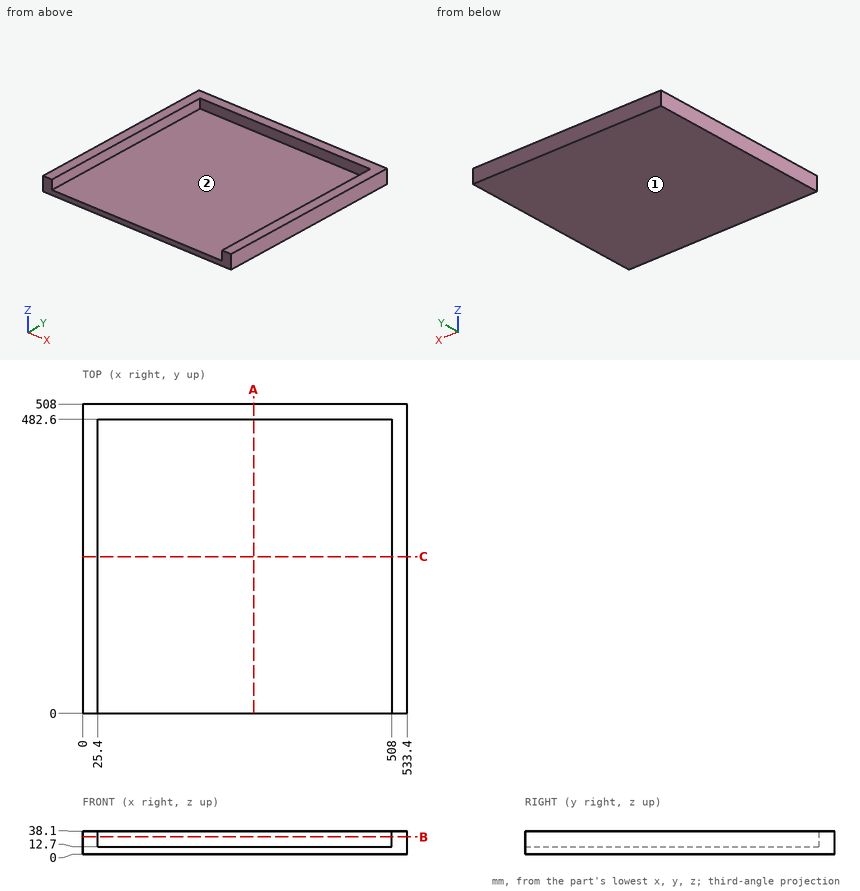
Here's the drawing with two shaded views (mm, measured from the low corner). I have some questions. Coordinates: 2 decimals unless noted, no trailing zeros. Write each loop counter-clockwise with the first axis right and the second up, starting at its lowest first coordinate (ties: lowest second). Pieces come first, ordered by that corner, then holes. Notation, with made-up numbers: (57.25, 67.25) -> (67.25, 67.25) arc R4 cw to (67.25, 71.25) -> close; hole circle Ø11 at (17, 79). An arc over 180 degrees is marked (long way). Answer as CSV lines item,"result".
1) If we section it at A-A on x = 281: Please give me the cut outline in (y, z), then the cut area to 3 significant figures.
Check result:
outline,"(0, 0) -> (508, 0) -> (508, 38.1) -> (482.6, 38.1) -> (482.6, 12.7) -> (0, 12.7) -> close"
area,"7,100 mm²"
2) If I drill on line 1 (X direction, y = 461.5, z = 28.5); line 2 (Z direction, x = 501.5, y = 338.5); line 3 (Y direction, x = 246, z = 21), over which ranges is the centre line in solid material (lowest first)? Write a range as from..to.
Check result:
line 1,"0..25.4, 508..533.4"
line 2,"0..12.7"
line 3,"482.6..508"
3) Will these pins go through, and if not, where does the flat tip stop? P1, Ø8, axis at x = 182.5, y = 416.5, coming from the +Z side; P2, Ø7.5, axis at x = 351.5, z = 30, coming from the -Y side.
Check result:
P1,"z = 12.7"
P2,"y = 482.6"
4) If we section it at B-B on z = 29: Please give me the cut outline in (x, y).
Check result:
outline,"(0, 0) -> (25.4, 0) -> (25.4, 482.6) -> (508, 482.6) -> (508, 0) -> (533.4, 0) -> (533.4, 508) -> (0, 508) -> close"
5) If we section it at C-C on y = 257.5: Please give me the cut outline in (x, z).
Check result:
outline,"(0, 0) -> (533.4, 0) -> (533.4, 38.1) -> (508, 38.1) -> (508, 12.7) -> (25.4, 12.7) -> (25.4, 38.1) -> (0, 38.1) -> close"
6) If we mould it in two halves opening along X, with no side actions, what happens to the marked faces 1 and 2? For each: +X half, -X half, draft (parallel to the pull), parting line (faces both ways), or undercut.
Check result:
face 1,"draft"
face 2,"undercut"
